Input: part model. Units: mm. Frame: model coordinates. A direction names the side the tool comes from. Give positions to 0.01 mm unless a question says otherwise; leave off trailing zeros. Write each loop counter-clockwise with the first axis right and the second up, starting at its lowest first coordinate (ties: lowest second). Pieces come first, ordered by that corner, then holes. Notation, with made-up numbers: (-30, -36) - (12, -36) arc R28 cw to (12, -11) - close; hole circle Ø10 at (82.5, 85). An arc over 180 degrees is marked (long way). Answer as CSV lines item,"result".
```python
from build123d import *

# Parameters (mm, degrees)
BOSS_EXTRU_1_DEPTH = 10
ESQUISSE3_W        = 3
ESQUISSE3_H        = 10
BOSS_EXTRU_2_DEPTH = 40


with BuildPart() as part:
    # Esquisse2 → Boss.-Extru.1 (new body)
    with BuildSketch(Plane(origin=(0, 0, 0), x_dir=(1, 0, 0), z_dir=(0, 1, 0))):
        with BuildLine():
            Line((0, 71.5), (0, 68.5))
            ThreePointArc((0, 68.5), (48.436814511, 48.436814511), (68.5, 0))
            ThreePointArc((68.5, 0), (48.436814511, -48.436814511), (0, -68.5))
            Line((0, -68.5), (0, -71.5))
            ThreePointArc((0, -71.5), (50.558134855, -50.558134855), (71.5, 0))
            ThreePointArc((71.5, 0), (50.558134855, 50.558134855), (0, 71.5))
        make_face()
    extrude(amount=BOSS_EXTRU_1_DEPTH)

    # Esquisse3 → Boss.-Extru.2 (add)
    with BuildSketch(Plane.ZY):
        with Locations((-70, 5)):
            Rectangle(ESQUISSE3_W, ESQUISSE3_H)
        with Locations((70, 5)):
            Rectangle(ESQUISSE3_W, ESQUISSE3_H)
    extrude(amount=BOSS_EXTRU_2_DEPTH)


solid = part.part
```
Item 1: Cut plane D-D on z = -32. Return the cut outline in (x, y).
The answers:
outline,"(60.57, 0) - (63.94, 0) - (63.94, 10) - (60.57, 10) - close"
Item 2: Mould query, pull axis Z, two halves, no side actions, for faces 1 (the face through (-40, 5, 70)), 2 (the face through (-20, 5, -71.5)), 3 (the face through (-20, 5, 68.5)). Classes: +Z half, -Z half, draft (parallel to the pull), parting line (faces both ways), or undercut.
The answers:
face 1,"draft"
face 2,"-Z half"
face 3,"undercut"
Item 3: Cut plane C-C on x = 13. Return the cut outline in (y, z), plus the area to 3 significant figures.
The answers:
outline,"(0, -70.31) - (10, -70.31) - (10, -67.26) - (0, -67.26) - close; (0, 67.26) - (10, 67.26) - (10, 70.31) - (0, 70.31) - close"
area,"61.1 mm²"
Item 4: Contact query for flat-ended pins moving along their axis: pin 1 (6 mm diameter, centred on x = 35, y = 4, fed in from -Z); pin 2 (3 mm diameter, centred on x = 48, z = 47, fed in from -Y); pin 3 (5 mm diameter, centred on x = 44.5, y = 7, fed in from +Z); pin 4 (1.5 mm diameter, centred on y = 4.5, z = 5.5, fed in from +X). Output: stop coordinate, or through.
The answers:
pin 1,"z = -63.94"
pin 2,"y = 0"
pin 3,"z = 57.86"
pin 4,"x = 71.34"
Item 5: Cut plane B-B on y = 7.5. Return the cut outline in (x, z), plus the area to 3 significant figures.
The answers:
outline,"(-40, -71.5) - (0, -71.5) arc R71.5 ccw to (0, 71.5) - (-40, 71.5) - (-40, 68.5) - (0, 68.5) arc R68.5 cw to (0, -68.5) - (-40, -68.5) - close"
area,"900 mm²"
Item 6: Reachability of faces 4 (the face through (66, 10, 21)), 5 (the face through (-20, 5, -68.5)) from +Z, -Z, +X, -X, +Y, -Y: full face, straight path, thin tool, end or side. Return the list, or none.
The answers:
face 4,"+Z, -Z, +X, -X, +Y"
face 5,"-X, +Y, -Y"
Item 7: Ray query, line 1 (Z direction, x = -5, y = 4.75); line 2 (Z direction, x = 38.5, y = 8.5); line 3 (X direction, y = 5.5, z = -29). Return the intervals inside material, ascending. Write a range as from..to.
The answers:
line 1,"-71.5..-68.5, 68.5..71.5"
line 2,"-60.25..-56.66, 56.66..60.25"
line 3,"62.06..65.35"
Item 8: Cut plane A-A on x = -33. Return the cut outline in (y, z).
The answers:
outline,"(0, -71.5) - (10, -71.5) - (10, -68.5) - (0, -68.5) - close; (0, 68.5) - (10, 68.5) - (10, 71.5) - (0, 71.5) - close"
